The model under review builds one solid part; all positions refer to its coordinate system, in mm. Face numbers are marked on the shaded views. A direction names the side the tool comes from. Coordinates: 2 decimals unless noted, no trailing zeros. Write each loop counter-clockwise with the first axis right and the second up, starting at its lowest first coordinate (ties: lowest second). Pieces come first, ordered by that corner, then holes.
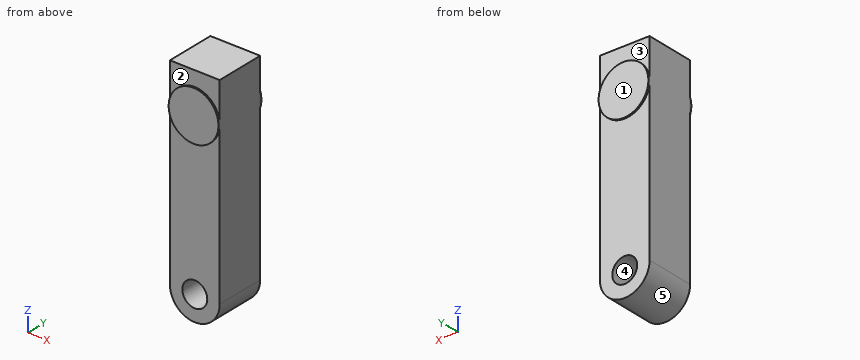
```python
from build123d import *

# Parameters (mm, degrees)
F1_DEPTH = 1.5875
F2_DEPTH = 1.6863590572


with BuildPart() as f1:
    # F0 (on Front) → F1 (new body, symmetric)
    with BuildSketch(Plane.XZ):
        with BuildLine():
            Line((-1.5875, 10.16), (-1.5875, 0))
            Line((-1.5875, 0), (-0.79375, 0))
            ThreePointArc((-0.79375, 0), (0, 0.79375), (0.79375, 0))
            Line((0.79375, 0), (1.5875, 0))
            Line((1.5875, 0), (1.5875, 10.16))
            ThreePointArc((1.5875, 10.16), (0, 8.5725), (-1.5875, 10.16))
        make_face()
        with BuildLine():
            ThreePointArc((1.5875, 10.16), (0, 11.7475), (-1.5875, 10.16))
            ThreePointArc((-1.5875, 10.16), (0, 8.5725), (1.5875, 10.16))
        make_face()
        with BuildLine():
            Line((-1.5875, 12.7), (-1.5875, 10.16))
            ThreePointArc((-1.5875, 10.16), (0, 11.7475), (1.5875, 10.16))
            Line((1.5875, 10.16), (1.5875, 12.7))
            Line((1.5875, 12.7), (-1.5875, 12.7))
        make_face()
        with BuildLine():
            Line((-0.79375, 0), (-1.5875, 0))
            ThreePointArc((-1.5875, 0), (0, -1.5875), (1.5875, 0))
            Line((1.5875, 0), (0.79375, 0))
            ThreePointArc((0.79375, 0), (0, -0.79375), (-0.79375, 0))
        make_face()
    extrude(amount=F1_DEPTH, both=True)

    # F0 (on Front) → F2 (join, symmetric)
    with BuildSketch(Plane.XZ):
        with BuildLine():
            ThreePointArc((1.5875, 10.16), (0, 11.7475), (-1.5875, 10.16))
            ThreePointArc((-1.5875, 10.16), (0, 8.5725), (1.5875, 10.16))
        make_face()
    extrude(amount=F2_DEPTH, both=True)


solid = f1.part
```
Item 1: Take a section at A-A, the plane x = 0. Write out the cut boundary in (y, z), plus the area to 3 significant figures.
Solved:
outline: (-1.69, 8.57) - (-1.59, 8.57) - (-1.59, 0.79) - (1.59, 0.79) - (1.59, 8.57) - (1.69, 8.57) - (1.69, 11.75) - (1.59, 11.75) - (1.59, 12.7) - (-1.59, 12.7) - (-1.59, 11.75) - (-1.69, 11.75) - close; (-1.59, -1.59) - (1.59, -1.59) - (1.59, -0.79) - (-1.59, -0.79) - close
area: 41.0 mm2
Item 2: Mouldability with a two-part tool opening along X and no side actions: class the marked faces 3, 4 and 5 as pulls with the +X half, pulls with the -X half, needs draft (parallel to the pull), parting line crosses it, or undercut.
Solved:
face 3: needs draft
face 4: undercut
face 5: parting line crosses it
Item 3: Take a section at B-B, the plane y = 0.55. Write out the cut boundary in (x, z) (1 decimal).
Solved:
outline: (-1.6, 0) arc R1.6 ccw to (1.6, 0) - (1.6, 12.7) - (-1.6, 12.7) - close; hole circle Ø1.6 at (0, 0)
Item 4: For pin 1 (1 mm diameter, centred on x = 0.5, z = 6, fed in from +Y), flat-tipped, find the tip position at first contact; note if it passes through.
Solved:
pin 1: stops at y = 1.59
Item 5: To check wall thickness, follow line 1 along Z through (x, y) = (0, 0.55); line 2 along X through (y, z) = (-0.7, 0); line 3 along Z through (x, y) = (0.6, 0). State the ranges of each line that lie inside material, in increasing order.
Solved:
line 1: z = -1.59 to -0.79, 0.79 to 12.7
line 2: x = -1.59 to -0.79, 0.79 to 1.59
line 3: z = -1.47 to -0.52, 0.52 to 12.7
Item 6: Take a section at C-C, the plane x = -1.2. Write out the cut boundary in (y, z).
Solved:
outline: (-1.69, 9.12) - (-1.59, 9.12) - (-1.59, -1.04) - (1.59, -1.04) - (1.59, 9.12) - (1.69, 9.12) - (1.69, 11.2) - (1.59, 11.2) - (1.59, 12.7) - (-1.59, 12.7) - (-1.59, 11.2) - (-1.69, 11.2) - close
Item 7: Machinability: for the marked faces 1 and 2, which of the approach directions +Z, -Z, +X, -X, +Y, -Y give a long, thin tool a straight path to every point of the face, cutting with its end or side? Answer none if there is none.
Solved:
face 1: +Z, -Z, +X, -X, +Y
face 2: +Z, -Y
Item 8: Take a section at D-D, the plane x = 0.65. Write out the cut boundary in (y, z), plus the area to 3 significant figures.
Solved:
outline: (-1.69, 8.71) - (-1.59, 8.71) - (-1.59, 0.46) - (1.59, 0.46) - (1.59, 8.71) - (1.69, 8.71) - (1.69, 11.61) - (1.59, 11.61) - (1.59, 12.7) - (-1.59, 12.7) - (-1.59, 11.61) - (-1.69, 11.61) - close; (-1.59, -1.45) - (1.59, -1.45) - (1.59, -0.46) - (-1.59, -0.46) - close
area: 42.6 mm2
